Read the model definition and answer for the solid it produces. Units are mm, in the model's axes. A direction names the side the tool comes from. Give positions to 0.01 mm unless a question says otherwise; leave off trailing zeros. Write each loop counter-clockwise with the first axis right and the second up, starting at its lowest first coordinate (ties: lowest second). Pieces come first, ordered by that corner, then holes. Notation, with made-up numbers: (3, 65) - (57, 65) arc R24 ccw to (57, 91) - close; hole circle Ø9 at (81.25, 68.5). An arc over 180 degrees is marked (long way). Answer as CSV lines item,"result".
```python
from build123d import *

# Parameters (mm, degrees)
F0_R     = 150
F1_DEPTH = 70
F2_W     = 70
F2_H     = 3
F3_DEPTH = 196.784
F4_R     = 9.5
F5_DEPTH = 184


with BuildPart() as f1:
    # F0 (on Right) → F1 (new body)
    with BuildSketch(Plane.YZ):
        Circle(F0_R)
    extrude(amount=F1_DEPTH)

    # F2 (on Front) → F3 (join)
    with BuildSketch(Plane.XZ):
        with Locations((35, -81.733)):
            Rectangle(F2_W, F2_H)
    extrude(amount=F3_DEPTH)

    # F4 (on face) → F5 (cut)
    with BuildSketch(Plane.YZ.offset(70)):
        Circle(F4_R)
    extrude(amount=-F5_DEPTH, mode=Mode.SUBTRACT)


solid = f1.part
```
(1) A cutting plane is placed at B-B (x = 19.5). Write down the section's boundary in (y, z), and give its area (3 significant figures).
Worked out:
outline,"(-196.78, -83.23) - (-124.79, -83.23) arc R150 ccw (long way) to (-126.74, -80.23) - (-196.78, -80.23) - close; hole circle Ø19 at (0, 0)"
area,"70,600 mm^2"
(2) A cutting plane is placed at D-D (y = 68). Write down the section's boundary in (x, z).
Worked out:
outline,"(0, -133.7) - (70, -133.7) - (70, 133.7) - (0, 133.7) - close"
(3) Find the intervals of material crossed by L1, parallel to Z at x = 23, y = 0; L2, parallel to Z at x = 19, y = 6; L3, parallel to Y at x = 41, z = 18.5, in increasing order.
Worked out:
L1,"z = -150 to -9.5, 9.5 to 150"
L2,"z = -149.88 to -7.37, 7.37 to 149.88"
L3,"y = -148.85 to 148.85"
(4) The mould has two halves that part along Y. Classify faces 3 (the flat face through (35, -160, -83.233)), 4 (the cylindrical face through (35.49, 4.38, -8.43)): +Y half, -Y half, draft (parallel to the pull), parting line (faces both ways), or undercut.
Worked out:
face 3,"draft"
face 4,"undercut"
(5) A cutting plane is placed at A-A (y = 0). Write down the section's boundary in (x, z).
Worked out:
outline,"(0, -150) - (70, -150) - (70, -9.5) - (0, -9.5) - close; (0, 9.5) - (70, 9.5) - (70, 150) - (0, 150) - close"
(6) For faces 1 (the flat face through (35, -161, -80.233)), 2 (the flat face through (70, 13, 2)), determine the directions among +Z, -Z, +X, -X, +Y, -Y from which every point of the face is accessible in a straight line to the end or side of a thin tool.
Worked out:
face 1,"+X, -X, -Y"
face 2,"+Z, -Z, +X, +Y, -Y"
(7) Each of these flat-tipped pins is pushed along its axis until it touches: P1, Ø12, axis at x = 22, z = 120, coming from the -Y side; P2, Ø1, axis at x = 19.5, z = -29, coming from the -Y side; P3, Ø3, axis at x = 8, y = 9, coming from the -Z side; P4, Ø5, axis at y = 11, z = -114, coming from the -X side. Where does it stop, or does it pass through?
Worked out:
P1,"stops at y = -97.49"
P2,"stops at y = -147.27"
P3,"stops at z = -149.81"
P4,"stops at x = 0"
(8) A cutting plane is placed at C-C (z = 131.5). Write down the section's boundary in (x, y), and give its area (3 significant figures).
Worked out:
outline,"(0, -72.16) - (70, -72.16) - (70, 72.16) - (0, 72.16) - close"
area,"10,100 mm^2"
